Verification items for the finished model (mm, model axes). A direction names the side the tool comes from. Coordinates: 2 decimals unless noted, no trailing zeros. Write each loop counter-clockwise with the first axis right and the second up, starting at its lowest first coordinate (ties: lowest second). Pieces come first, ordered by that corner, then holes. Notation, with made-up numbers: (26, 79) - (51, 79) arc R33 cw to (51, 117) - close; hole circle Ø9 at (-27, 75.5). An arc over 180 degrees is marked (long way). Answer as CSV lines item,"result". Start each with the question number.
```python
from build123d import *

# Parameters (mm, degrees)
SKETCH2_W           = 44.45
SKETCH2_H           = 19.05
BOSS_EXTRUDE1_DEPTH = 12.7
SKETCH3_W           = 50.8
SKETCH3_H           = 25.4
BOSS_EXTRUDE2_DEPTH = 3.175
BOSS_EXTRUDE3_DEPTH = 25.4
SKETCH5_R           = 11.1125
CUT_EXTRUDE1_DEPTH  = 7.366
SKETCH6_R           = 3.2639
CUT_EXTRUDE2_DEPTH  = 50.098929275


with BuildPart() as part:
    # Sketch2 → Boss-Extrude1 (new body)
    with BuildSketch(Plane(origin=(0, 0, 0), x_dir=(1, 0, 0), z_dir=(0, 1, 0))):
        Rectangle(SKETCH2_W, SKETCH2_H)
    extrude(amount=-BOSS_EXTRUDE1_DEPTH)

    # Sketch3 → Boss-Extrude2 (add)
    with BuildSketch(Plane(origin=(0, 0, 0), x_dir=(1, 0, 0), z_dir=(0, 1, 0))):
        Rectangle(SKETCH3_W, SKETCH3_H)
    extrude(amount=BOSS_EXTRUDE2_DEPTH)

    # Sketch4 → Boss-Extrude3 (add, symmetric)
    with BuildSketch(Plane(origin=(0, 0, 0), x_dir=(0, 0, -1), z_dir=(1, 0, 0))):
        Polygon((-12.7, 3.175), (-12.7, 4.7625), (3.175, 19.05), (12.7, 19.05), (12.7, 3.175), align=None)
    extrude(amount=BOSS_EXTRUDE3_DEPTH, both=True)

    # Sketch5 → Cut-Extrude1 (cut)
    with BuildSketch(Plane(origin=(25.4, 0, 0), x_dir=(0, 0, -1), z_dir=(1, 0, 0))):
        with Locations((7.9375, 12.7)):
            Circle(SKETCH5_R)
    cut_extrude1 = extrude(amount=-CUT_EXTRUDE1_DEPTH, mode=Mode.SUBTRACT)

    # Sketch6 → Cut-Extrude2 (cut, through all)
    with BuildSketch(Plane(origin=(18.034, 0, 0), x_dir=(0, 0, -1), z_dir=(1, 0, 0))):
        with Locations((7.9375, 12.7)):
            Circle(SKETCH6_R)
    extrude(amount=-CUT_EXTRUDE2_DEPTH, mode=Mode.SUBTRACT)

    # Mirror1: Cut-Extrude1 across plane
    add(cut_extrude1.mirror(Plane(origin=(0, 0, 0), x_dir=(0, 0, 1), z_dir=(1, 0, 0))), mode=Mode.SUBTRACT)


solid = part.part
```
1. Scan lines: line 1 along X through (y, z) = (-6.5, 1.25) (3 decimals); line 2 along Z through (x, y) = (16, -4) (3 decimals); line 3 along Z through (x, y) = (-7, 12). Record each from-to range of solid material in increasing order. Write a range as from..to.
2. Cross-section at C-C (y = 12.7). Record the cut outline in (x, z) (3 decimals).
3. Draft check along Z on faces 1 (the face through (21.77, 3.58, -1.59)), 2 (the face through (0.36, 11.81, 4.87)), 3 (the face through (-25.4, 4, 3)), 4 (the face through (0, -6, -9.525)). Enter one of: pulls with the +Z half, pulls with the -Z half, needs draft (parallel to the pull), parting line crosses it, or undercut.
4. Depth check by flat-ended pin: P1, Ø10, axis at y = -7.5, z = -3, coming from the -X side (3 decimals); P2, Ø12.5, axis at y = 14.5, z = -4.5, coming from the -X side; P3, Ø8, axis at y = 12.5, z = -4, coming from the +X side; P4, Ø12, axis at y = -1, z = 2, coming from the -X side. Enter the tip coordinate at first touch or a pass-through.
5. Cross-section at B-B (z = 4.75). Record the cut outline in (x, y) (1 decimal), and give its area (3 significant figures).
6. Cross-section at D-D (y = -7). Record the cut outline in (x, z) (3 decimals), and give its area (3 significant figures).
7. Access from +Z, -Z, +X, -X, +Y, -Y to the whole of each face (thin tool, end or side, straight path). Record for faces 5 (the face through (-22.225, -6, 0)), 6 (the face through (0, 19.05, -8)), 7 (the face through (22.225, -6, 0)), 8 (the face through (0, -6, 9.525)).
Completed:
1,line 1,"x = -22.225..22.225"
1,line 2,"z = -9.525..9.525"
1,line 3,"z = -12.7..-11.13, -4.75..4.66"
2,outline,"(-25.4, 3.175) - (-18.034, 3.175) - (-18.034, -4.674) - (18.034, -4.674) - (18.034, 3.175) - (25.4, 3.175) - (25.4, 3.881) - (-25.4, 3.881) - close; (-18.034, -12.7) - (18.034, -12.7) - (18.034, -11.201) - (-18.034, -11.201) - close"
3,face 1,"undercut"
3,face 2,"pulls with the +Z half"
3,face 3,"needs draft"
3,face 4,"pulls with the -Z half"
4,P1,"stops at x = -22.225"
4,P2,"stops at x = -18.03"
4,P3,"stops at x = 18.03"
4,P4,"stops at x = -25.4"
5,outline,"(-25.4, 0) - (-22.2, 0) - (-22.2, -12.7) - (22.2, -12.7) - (22.2, 0) - (25.4, 0) - (25.4, 11.9) - (-25.4, 11.9) - close"
5,area,"1,170 mm2"
6,outline,"(-22.225, -9.525) - (22.225, -9.525) - (22.225, 9.525) - (-22.225, 9.525) - close"
6,area,"847 mm2"
7,face 5,"+Z, -Z, -X, -Y"
7,face 6,"+Z, -Z, +X, -X, +Y"
7,face 7,"+Z, -Z, +X, -Y"
7,face 8,"+Z, +X, -X, -Y"
